Here's how the part is built. I have some questions about the finished solid (model axes, mm). Face numbers are marked on the shaded views. A direction names the side the tool comes from. Coordinates: 2 decimals unless noted, no trailing zeros. Loops run counter-clockwise (first coordinate to the right, second up) from the corner with the lowest first, then second, coordinate; pieces in that order, holes last. Notation, with made-up numbers: (49.5, -2.75) -> (107.5, -2.75) arc R32 cw to (107.5, 34.25) -> close; hole circle Ø9 at (70, 61.5). An arc over 180 degrees is marked (long way). Answer as a JSON object with one key per item and string values. Group by question number.
1) If we mould it in two halves opening along X, with no side actions, what happens to the marked faces 3, 4 and 5? For each: +X half, -X half, draft (parallel to the pull), parting line (faces both ways), or undercut.
2) I want a section at A-A (y = -2.75). Write out the boundary of the cut face in (x, z), then the cut area to 3 significant figures.
3) Which directions (+Z, -Z, +X, -X, +Y, -Y) give clear straight access to the entire face, cutting with the end or side of a thin tool? Please do the marked faces 1 and 2.
4) I need wall thicknesses on probe 1 along X at (y, z) = (0.3, 2.5); probe 2 along Z at (x, y) = (8.5, -0.75); probe 3 along Z at (x, y) = (-4.5, -0.5). Which ranges of each line are inside material? Lowest first, please. Write a range as [from, to].
5) I want a section at D-D (x = -7.5). Write out the boundary of the cut face in (y, z).
6) I'm going to push flat-ended pins straight in: pin 1 (1.5 mm diameter, centred on x = -4.5, z = -0.5, fed in from -Y); pin 2 (1.4 mm diameter, centred on x = -2.5, z = 2.5, fed in from -Y). Where does each tip first touch, or does it pass through?
7) I want a section at B-B (x = 5). Write out the boundary of the cut face in (y, z), then the cut area to 3 significant figures.
```python
from build123d import *

# Parameters (mm, degrees)
SKETCH1_R           = 1.5
SKETCH1_R_2         = 0.75
BOSS_EXTRUDE1_DEPTH = 2
SKETCH1_3_W         = 20
SKETCH1_3_H         = 10
BOSS_EXTRUDE2_DEPTH = 1
SKETCH1_4_R         = 0.75
CUT_EXTRUDE1_DEPTH  = 1
SKETCH1_5_W         = 20
SKETCH1_5_H         = 10
SKETCH1_5_W_2       = 18
SKETCH1_5_H_2       = 8
SKETCH1_5_R         = 2.035533906
SKETCH1_5_R_2       = 1.5
BOSS_EXTRUDE3_DEPTH = 5


with BuildPart() as part:
    # Sketch1 → Boss-Extrude1 (new body)
    with BuildSketch(Plane(origin=(0, 0, 0), x_dir=(1, 0, 0), z_dir=(0, 1, 0))):
        with Locations(Location((-7.5, 2.5, 0), (0, 0, 270))):
            Circle(SKETCH1_R)
        with Locations(Location((-2.5, 2.5, 0), (0, 0, 270))):
            Circle(SKETCH1_R)
        with Locations(Location((2.5, 2.5, 0), (0, 0, 270))):
            Circle(SKETCH1_R)
        with Locations(Location((7.5, 2.5, 0), (0, 0, 270))):
            Circle(SKETCH1_R)
        with Locations(Location((7.5, -2.5, 0), (0, 0, 270))):
            Circle(SKETCH1_R)
        with Locations(Location((2.5, -2.5, 0), (0, 0, 270))):
            Circle(SKETCH1_R)
        with Locations(Location((-2.5, -2.5, 0), (0, 0, 270))):
            Circle(SKETCH1_R)
        with Locations(Location((-7.5, -2.5, 0), (0, 0, 270))):
            Circle(SKETCH1_R)
        with Locations((-7.5, 2.5)):
            Circle(SKETCH1_R_2)
        with Locations((-2.5, 2.5)):
            Circle(SKETCH1_R_2)
        with Locations((2.5, 2.5)):
            Circle(SKETCH1_R_2)
        with Locations((7.5, 2.5)):
            Circle(SKETCH1_R_2)
        with Locations((7.5, -2.5)):
            Circle(SKETCH1_R_2)
        with Locations((2.5, -2.5)):
            Circle(SKETCH1_R_2)
        with Locations((-2.5, -2.5)):
            Circle(SKETCH1_R_2)
        with Locations((-7.5, -2.5)):
            Circle(SKETCH1_R_2)
    extrude(amount=BOSS_EXTRUDE1_DEPTH)

    # Sketch1_3 → Boss-Extrude2 (add)
    with BuildSketch(Plane(origin=(0, 0, 0), x_dir=(1, 0, 0), z_dir=(0, 1, 0))):
        Rectangle(SKETCH1_3_W, SKETCH1_3_H)
    extrude(amount=BOSS_EXTRUDE2_DEPTH)

    # Sketch1_4 → Cut-Extrude1 (cut)
    with BuildSketch(Plane(origin=(0, 0, 0), x_dir=(1, 0, 0), z_dir=(0, 1, 0))):
        with Locations(Location((-7.5, -2.5, 0), (0, 0, 270))):
            Circle(SKETCH1_4_R)
        with Locations(Location((-2.5, -2.5, 0), (0, 0, 270))):
            Circle(SKETCH1_4_R)
        with Locations(Location((2.5, -2.5, 0), (0, 0, 270))):
            Circle(SKETCH1_4_R)
        with Locations(Location((7.5, -2.5, 0), (0, 0, 270))):
            Circle(SKETCH1_4_R)
        with Locations(Location((7.5, 2.5, 0), (0, 0, 270))):
            Circle(SKETCH1_4_R)
        with Locations(Location((2.5, 2.5, 0), (0, 0, 270))):
            Circle(SKETCH1_4_R)
        with Locations(Location((-2.5, 2.5, 0), (0, 0, 270))):
            Circle(SKETCH1_4_R)
        with Locations(Location((-7.5, 2.5, 0), (0, 0, 270))):
            Circle(SKETCH1_4_R)
    extrude(amount=CUT_EXTRUDE1_DEPTH, mode=Mode.SUBTRACT)

    # Sketch1_5 → Boss-Extrude3 (add)
    with BuildSketch(Plane(origin=(0, 0, 0), x_dir=(1, 0, 0), z_dir=(0, 1, 0))):
        Rectangle(SKETCH1_5_W, SKETCH1_5_H)
        Rectangle(SKETCH1_5_W_2, SKETCH1_5_H_2, mode=Mode.SUBTRACT)
        with Locations(Location((-5, 0, 0), (0, 0, 270))):
            Circle(SKETCH1_5_R)
        with Locations(Location((-5, 0, 0), (0, 0, 270))):
            Circle(SKETCH1_5_R_2, mode=Mode.SUBTRACT)
        with Locations(Location((0, 0, 0), (0, 0, 270))):
            Circle(SKETCH1_5_R)
        with Locations(Location((0, 0, 0), (0, 0, 270))):
            Circle(SKETCH1_5_R_2, mode=Mode.SUBTRACT)
        with Locations(Location((5, 0, 0), (0, 0, 270))):
            Circle(SKETCH1_5_R)
        with Locations(Location((5, 0, 0), (0, 0, 270))):
            Circle(SKETCH1_5_R_2, mode=Mode.SUBTRACT)
    extrude(amount=-BOSS_EXTRUDE3_DEPTH)


solid = part.part
```
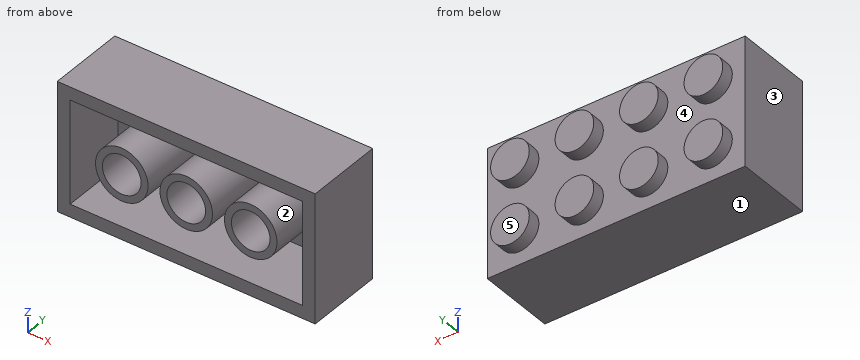
Determined:
{
 "1": {"face 3": "-X half", "face 4": "undercut", "face 5": "draft"},
 "2": {"outline": "(-10, -5) -> (10, -5) -> (10, 5) -> (-10, 5) -> close; circle Ø4.07 at (-5, 0); circle Ø4.07 at (0, 0); circle Ø4.07 at (5, 0); hole (-9, -4) -> (9, -4) -> (9, 4) -> (-9, 4) -> close; hole circle Ø3 at (-5, 0); hole circle Ø3 at (0, 0); hole circle Ø3 at (5, 0)", "area": "73.8 mm^2"},
 "3": {"face 1": "-Z, +X, -X, +Y, -Y", "face 2": "-Y"},
 "4": {"probe 1": "[-10, -8.25], [-6.75, -3.25], [-1.75, 1.75], [3.25, 6.75], [8.25, 10]", "probe 2": "[-5, -4], [4, 5]", "probe 3": "[-5, -4], [-1.97, -1.41], [1.41, 1.97], [4, 5]"},
 "5": {"outline": "(-5, -5) -> (1, -5) -> (1, -4) -> (2, -4) -> (2, -1) -> (1, -1) -> (1, 1) -> (2, 1) -> (2, 4) -> (1, 4) -> (1, 5) -> (-5, 5) -> (-5, 4) -> (0, 4) -> (0, 3.25) -> (1, 3.25) -> (1, 1.75) -> (0, 1.75) -> (0, -1.75) -> (1, -1.75) -> (1, -3.25) -> (0, -3.25) -> (0, -4) -> (-5, -4) -> close"},
 "6": {"pin 1": "y = 0", "pin 2": "y = 1"},
 "7": {"outline": "(-5, -5) -> (1, -5) -> (1, 5) -> (-5, 5) -> (-5, 4) -> (0, 4) -> (0, 2.04) -> (-5, 2.04) -> (-5, 1.5) -> (0, 1.5) -> (0, -1.5) -> (-5, -1.5) -> (-5, -2.04) -> (0, -2.04) -> (0, -4) -> (-5, -4) -> close", "area": "25.4 mm^2"}
}
